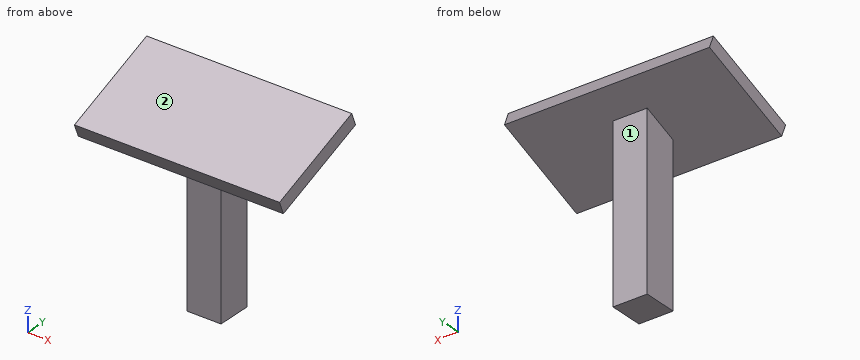
from build123d import *

# Parameters (mm, degrees)
F0_W     = 152.4
F0_H     = 152.4
F1_DEPTH = 762
F3_DEPTH = 152.401
F4_W     = 914.4
F4_H     = 457.2
F5_DEPTH = 60.96


with BuildPart() as f1:
    # F0 (on Top) → F1 (new body)
    with BuildSketch(Plane.XY):
        with Locations((7.154546032, -11.9188567623)):
            Rectangle(F0_W, F0_H)
    extrude(amount=F1_DEPTH)

    # F2 (on face) → F3 (cut, through all)
    with BuildSketch(Plane.YZ.offset(83.354546032)):
        Polygon((64.2811432377, 762), (-88.1188567623, 762), (-88.1188567623, 701.04), align=None)
    extrude(amount=-F3_DEPTH, mode=Mode.SUBTRACT)

    # F4 (on face) → F5 (join)
    with BuildSketch(Plane(origin=(0, -253.8922561052, 634.7306402629), x_dir=(1, 0, 0), z_dir=(0, -0.3713906764, 0.9284766909))):
        with Locations((7.154546032, 260.6133268807)):
            Rectangle(F4_W, F4_H)
    extrude(amount=F5_DEPTH)


solid = f1.part
The model under review builds one solid part; all positions refer to its coordinate system, in mm. Face numbers are marked on the shaded views. A direction names the side the tool comes from. Give positions to 0.01 mm unless a question says otherwise; leave off trailing zeros. Order: outer loops, then holes, each group sorted by start corner. A loop starts at its lowest first (then second) coordinate and runs counter-clockwise, first axis right, second up. Notation, with made-up numbers: M -28,82.5 L 20,82.5 A29 cw 20,102.5 Z; hole C 21,33 d3. An arc over 180 degrees is marked long. Use one line per item in the form item = value. Start each with the question number.
Item 1: We need section B-B on z = 492. Give the boundary of the cut face in (x, y), plus the area to 3 significant figures.
Item 2: Insertion check: pin 1 Ø5 at (y, z) = (-38.5, 419.5) entering from -X; pin 2 Ø4 at (x, y) = (-74.5, -41.5) entering from -Z; pin 3 Ø8 at (x, z) = (-241, 777.5) entering from -Y. Each pin has a flat end and moves straight along its axis. Give the tip position at first contact, or say it passes through.
Item 3: We need section D-D on z = 735.5. Give the boundary of the cut face in (x, y), plus the area to 3 significant figures.
Item 4: For the marked faces 1 and 2, list the 3-axis set-ups (+Z, -Z, +X, -X, +Y, -Y) from which the entire face can be reached by the end or side of a thin tool; tool diameter is ignored.
Item 5: We need section A-A on x = 20.5. Give the boundary of the cut face in (y, z).
Item 6: We need section C-C on y = -142. Give the boundary of the cut face in (x, z).
Item 7: To check wall thickness, follow line 1 along X through (y, z) = (37, 578); line 2 along Y through (x, z) = (-50, 81); line 3 along Y through (x, z) = (245.5, 797). State the ranges of each line that lie inside material, in increasing order. Write a range as from..to.
Completed:
q1.outline = M -69.05,-88.12 L 83.35,-88.12 L 83.35,64.28 L -69.05,64.28 Z
q1.area = 23,200 mm²
q2.pin_1 = -69.05
q2.pin_2 = 718.89
q2.pin_3 = -71.11
q3.outline = M -450.05,-166.11 L 464.35,-166.11 L 464.35,-1.97 L 83.35,-1.97 L 83.35,64.28 L -69.05,64.28 L -69.05,-1.97 L -450.05,-1.97 Z
q3.area = 160,000 mm²
q4.face_1 = -Z, +X, -X, +Y
q4.face_2 = +Z, +X, -X, -Y
q5.outline = M -246.81,703.22 L -224.17,646.62 L -88.12,701.04 L -88.12,0 L 64.28,0 L 64.28,762 L 200.33,816.42 L 177.69,873.02 Z
q6.outline = M -450.05,679.49 L 464.35,679.49 L 464.35,745.14 L -450.05,745.14 Z
q7.line_1 = -69.05..83.35
q7.line_2 = -88.12..64.28
q7.line_3 = -12.36..151.78
